The figure shows three views and two pictorial views of one solid part (mm, origin at its lowest corner). Answer the questions. A direction names the side the tool comes from. Round coordinates to 2 decimals unless told otherwise and drop trailing zeros. Order: outer loops, then holes, each group sorted by start corner. A loop starts at its lowest first (then second) coordinate and runs counter-clockwise, first axis right, second up.
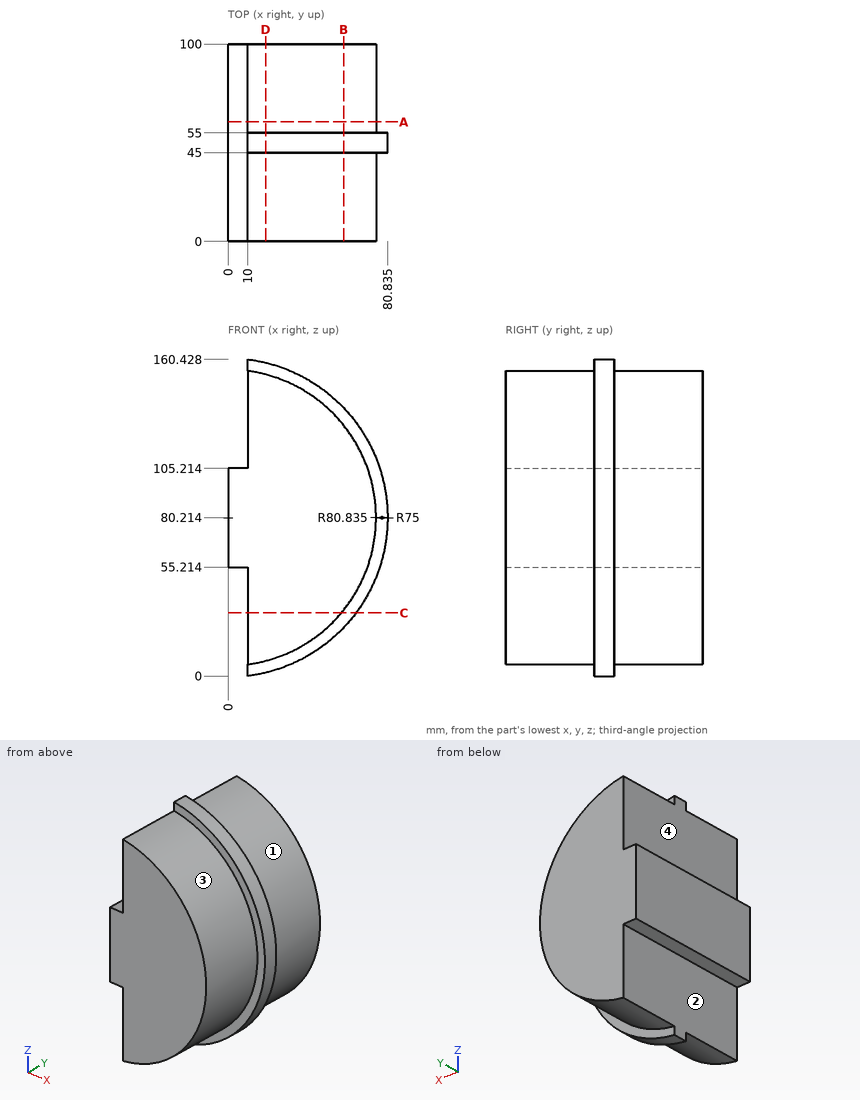
Item 1: Find section C-C (z = 32). Write down the section's boundary in (x, y).
Item 2: Find the intervals of material crossed by line 1 along Z through (x, y) = (5.5, 51); line 2 along X through (y, z) = (61.5, 37); line 3 along X through (y, z) = (60, 106), in increasing order.
Item 3: A tool of negligible diameter and unlimited length cuts with its end or side. For the marked faces 1, 2, 3 and 4, from which of +Z, -Z, +X, -X, +Y, -Y can it reach the whole face along a straight path? Write none if from no direction.
Item 4: Find section A-A (y = 60.5). Write down the section's boundary in (x, z).
Item 5: Given pin 1 (6 mm diameter, centred on y = 69, z = 89, fed in from +X); pin 2 (8 mm diameter, centred on x = 7.5, y = 67.5, fed in from +Z); pin 3 (16.5 mm diameter, centred on y = 43.5, z = 144.5, fed in from -X), each flat-ended and moving along its own axis, determine where each tip first touches the part or whether it passes through.
Item 6: Find section B-B (x = 58.5). Write down the section's boundary in (y, z).
Item 7: Find section D-D (x = 19). Write down the section's boundary in (y, z), plus the area to 3 significant figures.
Model answer:
1. outline: (10, 0) - (57.45, 0) - (57.45, 45) - (64.88, 45) - (64.88, 55) - (57.45, 55) - (57.45, 100) - (10, 100) - close
2. line 1: z = 55.21 to 105.21
2. line 2: x = 10 to 61.3
2. line 3: x = 10 to 70.43
3. face 1: +X, +Y
3. face 2: -Z, -X, +Y, -Y
3. face 3: +X, -Y
3. face 4: +Z, -X, +Y, -Y
4. outline: (0, 55.21) - (10, 55.21) - (10, 5.88) arc R75 ccw to (10, 154.54) - (10, 105.21) - (0, 105.21) - close
5. pin 1: stops at x = 74.78
5. pin 2: stops at z = 154.54
5. pin 3: stops at x = 10
6. outline: (0, 33.28) - (45, 33.28) - (45, 24.43) - (55, 24.43) - (55, 33.28) - (100, 33.28) - (100, 127.15) - (55, 127.15) - (55, 136) - (45, 136) - (45, 127.15) - (0, 127.15) - close
7. outline: (0, 7.66) - (45, 7.66) - (45, 1.64) - (55, 1.64) - (55, 7.66) - (100, 7.66) - (100, 152.77) - (55, 152.77) - (55, 158.78) - (45, 158.78) - (45, 152.77) - (0, 152.77) - close
7. area: 14,600 mm2
